For this review, use the dimensioned drawing (mm, ordinates from the lowest corner) and the shaded views. A direction names the side the tool comes from. Give positions to 0.01 mm unless a question says otherwise; leave off trailing zeros. Write each loop counter-clockwise with the first axis right and the second up, starting at its lowest first coordinate (ties: lowest second). Pieces come first, ordered by that corner, then holes. Notation, with made-up numbers: M 28.5,65.5 L 54.5,65.5 A31 cw 54.5,99.5 Z; hole C -5,87.25 d3. An arc over 180 degrees is marked long. One line per item, written item: value. Start each with the question number.
Item 1: Tool access review of the marked faces 4 and 5: name each direction out of +Z, -Z, +X, -X, +Y, -Y from which nothing blocks a thin tool from reaching the whole face with its end or side.
Item 2: Consider section C-C, the plane x = 2.5. Write out the cut boundary in (y, z).
Item 3: Consider section A-A, the plane y = 14. Write out the cut boundary in (x, z).
Item 4: Clearance check with flat-ended pins moving along their axes: pin 1 Ø4 at (x, y) = (7.5, 3) entering from -Z; pin 2 Ø13 at (y, z) = (14, 14) entering from -X; pin 3 Ø1 at (x, z) = (7, 17.5) entering from -Y. State where each tip first meets the part, or that it passes through.
Item 5: Consider section D-D, the plane y = 6. Write out the cut boundary in (x, z).
Item 6: Mouldability with a two-part tool opening along Y and no side actions: class the marked faces 1, 2 and 3 as released by +Y, released by -Y, zero draft, split by the parting line, or undercut.
Item 7: To check wall thickness, follow probe 1 along Y at (x, z) = (6.7, 14); probe 2 along Y at (x, z) = (1.2, 14); probe 3 along X at (y, z) = (25.25, 21). State the ranges of each line that lie inside material, in increasing order.
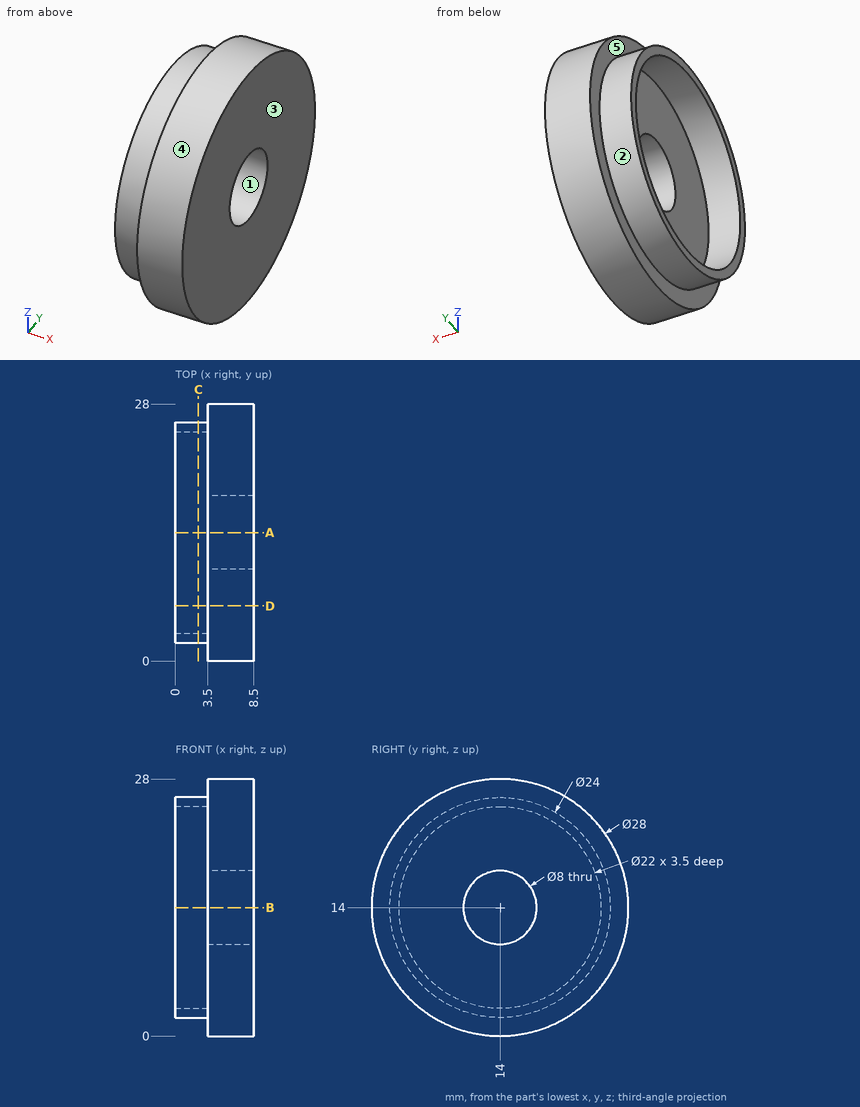
Model answer:
1. face 4: +X, -X
1. face 5: -X
2. outline: C 14,14 d24; hole C 14,14 d22
3. outline: M 0,2 L 3.5,2 L 3.5,0 L 8.5,0 L 8.5,10 L 3.5,10 L 3.5,3 L 0,3 Z; M 0,25 L 3.5,25 L 3.5,18 L 8.5,18 L 8.5,28 L 3.5,28 L 3.5,26 L 0,26 Z
4. pin 1: stops at z = 3.28
4. pin 2: stops at x = 3.5
4. pin 3: stops at y = 0.33
5. outline: M 0,5.06 L 3.5,5.06 L 3.5,2.51 L 8.5,2.51 L 8.5,25.49 L 3.5,25.49 L 3.5,22.94 L 0,22.94 L 0,21.55 L 3.5,21.55 L 3.5,6.45 L 0,6.45 Z
6. face 1: undercut
6. face 2: split by the parting line
6. face 3: zero draft
7. probe 1: y = 0 to 10, 18 to 28
7. probe 2: y = 2 to 3, 25 to 26
7. probe 3: x = 3.5 to 8.5
